```python
from build123d import *

# Parameters (mm, degrees)
SKETCH1_R             = 1.5
BASE_DEPTH            = 4
BATTERYCLIP_DEPTH     = 6
BOSS_EXTRUDE1_DEPTH   = 4
F_3_0MM_DOWEL_HOLE2_D = 3
CIRPATTERN2_COUNT     = 4
SKETCH7_R             = 10
REFRERENCE_DEPTH      = 10


with BuildPart() as part:
    # Sketch1 → Base (new body)
    with BuildSketch(Plane(origin=(0, 0, 0), x_dir=(1, 0, 0), z_dir=(0, 1, 0))):
        Polygon((100, 100), (65.656854249, 100), (20, 145.656854249), (20, 180), (0, 180), (0, 145.656854249), (-45.656854249, 100), (-80, 100), (-80, 80), (-45.656854249, 80), (0, 34.343145751), (0, 0), (20, 0), (20, 34.343145751), (65.656854249, 80), (100, 80), align=None)
        Polygon((51.514718626, 100), (20, 100), (20, 131.514718626), align=None, mode=Mode.SUBTRACT)
        Polygon((-31.514718626, 80), (0, 80), (0, 48.485281374), align=None, mode=Mode.SUBTRACT)
        Polygon((0, 131.514718626), (0, 100), (-31.514718626, 100), align=None, mode=Mode.SUBTRACT)
        Polygon((20, 48.485281374), (20, 80), (51.514718626, 80), align=None, mode=Mode.SUBTRACT)
        with Locations(Location((10, 90, 0), (0, 0, 270))):
            Circle(SKETCH1_R, mode=Mode.SUBTRACT)
    extrude(amount=BASE_DEPTH)

    # Sketch2 → BatteryClip (add)
    with BuildSketch(Plane(origin=(0, 4, 0), x_dir=(1, 0, 0), z_dir=(0, 1, 0))):
        Polygon((15.303300859, 50.402020254), (4.696699141, 39.795418536), (8.232233047, 36.25988463), (18.838834765, 46.866486348), align=None)
        Polygon((11.767766953, 143.74011537), (1.161165235, 133.133513652), (4.696699141, 129.597979746), (15.303300859, 140.204581464), align=None)
        Polygon((49.597979746, 84.696699141), (60.204581464, 95.303300859), (63.74011537, 91.767766953), (53.133513652, 81.161165235), align=None)
        Polygon((-43.74011537, 88.232233047), (-33.133513652, 98.838834765), (-29.597979746, 95.303300859), (-40.204581464, 84.696699141), align=None)
    extrude(amount=BATTERYCLIP_DEPTH)

    # Sketch6 → Boss-Extrude1 (add)
    with BuildSketch(Plane.XZ):
        Polygon((66.568542495, -160.710678119), (10, -104.142135624), (-46.568542495, -160.710678119), (-60.710678119, -146.568542495), (-4.142135624, -90), (-60.710678119, -33.431457505), (-46.568542495, -19.289321881), (10, -75.857864376), (66.568542495, -19.289321881), (80.710678119, -33.431457505), (24.142135624, -90), (80.710678119, -146.568542495), align=None)
    extrude(amount=-BOSS_EXTRUDE1_DEPTH)

    # Ø3.0mm Dowel Hole2 (through all)
    with Locations(Plane(origin=(5, 4, -5), x_dir=(0, 0, 1), z_dir=(0, 1, 0))):
        with Locations((0, 0), (-10, 0), (-10, 10), (0, 10), (-41.564971157, -10.150757595), (-55.707106781, -24.292893219), (-69.849242405, -38.435028843), (-28.431457505, -58.639610307), (-35.502525317, -51.568542495), (-28.431457505, -44.497474683), (-21.360389693, -51.568542495)):
            f_3_0mm_dowel_hole2 = Hole(F_3_0MM_DOWEL_HOLE2_D / 2)

    # CirPattern2: Ø3.0mm Dowel Hole2 ×4 about axis
    cirpattern2_axis = Axis((10, 0, -90), (0, 1, 0))
    for i in range(1, CIRPATTERN2_COUNT):
        add(f_3_0mm_dowel_hole2.rotate(cirpattern2_axis, i * 360 / CIRPATTERN2_COUNT), mode=Mode.SUBTRACT)

    # Sketch7 → Refrerence (cut)
    with BuildSketch(Plane(origin=(0, 4, 0), x_dir=(1, 0, 0), z_dir=(0, 1, 0))):
        with Locations(Location((10, 90, 0), (0, 0, 270))):
            Circle(SKETCH7_R)
    extrude(amount=-REFRERENCE_DEPTH, mode=Mode.SUBTRACT)


solid = part.part
```
Verification items for the finished model (mm, model axes). A direction names the side the tool comes from. Round coordinates to 2 decimals unless told otherwise and drop trailing zeros. Order: outer loops, then holes, each group sorted by start corner. A loop starts at its lowest first (then second) coordinate and runs counter-clockwise, first axis right, second up. Notation, with made-up numbers: (-25.75, -33) - (18.25, -33) arc R25 cw to (18.25, -7) - close; hole circle Ø4 at (29.25, 52). An arc over 180 degrees is marked (long way). Use CSV: the item, a comma, the result in double quotes.
(1) Gauge pin test, flat ends, axial feed: pin 1 Ø6 at (x, y) = (61.5, 4.5) entering from +Z; pin 2 Ø1.8 at (x, z) = (-19.29, -119.29) entering from -Y; pin 3 Ø1.2 at (y, z) = (1.5, -160.5) entering from +X; pin 4 Ø5 at (x, z) = (59.5, -146.57) entering from +Y. Record the tip position at first contact, or that the pin passes through.
Entries:
pin 1,"z = -21.4"
pin 2,"through"
pin 3,"x = 67.38"
pin 4,"y = 4"
(2) Section check A-A on y = 6. Record the boundary of the cut face in (x, z).
Entries:
outline,"(-43.74, -88.23) - (-33.13, -98.84) - (-29.6, -95.3) - (-40.2, -84.7) - close; (1.16, -133.13) - (11.77, -143.74) - (15.3, -140.2) - (4.7, -129.6) - close; (4.7, -39.8) - (15.3, -50.4) - (18.84, -46.87) - (8.23, -36.26) - close; (49.6, -84.7) - (60.2, -95.3) - (63.74, -91.77) - (53.13, -81.16) - close"
(3) Access from +Z, -Z, +X, -X, +Y, -Y to the whole of each face (thin tool, end or side, straight path). Record for faces 4 (the face through (13.46, 6.96, -41.49)), 5 (the face through (-45.09, 1.97, -49.05)), 6 (the face through (20, 2, -163)).
Entries:
face 4,"+Z, +X, +Y"
face 5,"-X, +Y, -Y"
face 6,"-Z, +Y, -Y"
(4) Mould release check, pull along Z, two halves, no side actions. Record for faces 1 (the face through (57.668, 1.972, -72.011)), 2 (the face through (27.768, 1.972, -42.112)), 3 (the face through (11, 0, -69)): released by +Z, released by -Z, zero draft, split by the parting line, or undercut.
Entries:
face 1,"undercut"
face 2,"released by +Z"
face 3,"zero draft"
(5) Thickness scan on probe 1 along Z at (x, y) = (10.5, 0.5); probe 2 along Z at (x, y) = (-3, 3.5); probe 3 along Z at (x, y) = (-6, 3.75). Record the ranges inside material, lowest first. Write a range as from..to.
Entries:
probe 1,"-180..-99.99, -80.01..0"
probe 2,"-142.66..-128.51, -117.14..-62.86, -51.49..-37.34"
probe 3,"-139.66..-134.67, -132.2..-125.51, -120.14..-59.86, -54.49..-47.8, -45.33..-40.34"
